Geometry: see drawing. Coordinates: mm, zero at the bounding-box minimum. Coordinates: 2 decimals unless noted, no trailing zeros. Write each loop counter-clockwise with the first axis right and the second up, starting at its lowest first coordinate (ties: lowest second). Pieces come first, ordered by that corner, then holes.
1) Section query A-A (x = 62.5). Output: boundary loops of the cut face in (y, z), then the cut area to 3 significant figures.
2) Section query B-B (y = 1.3). Output: boundary loops of the cut face in (x, z), then the cut area to 3 significant figures.
3) Line query: L1, parallel to Z at x = 89.5, y = 1.2; L2, parallel to X at y = 2.4, z = 71.5; L3, parallel to X at y = 3.95, z = 7.5. Output: solid intervals per line, ascending.
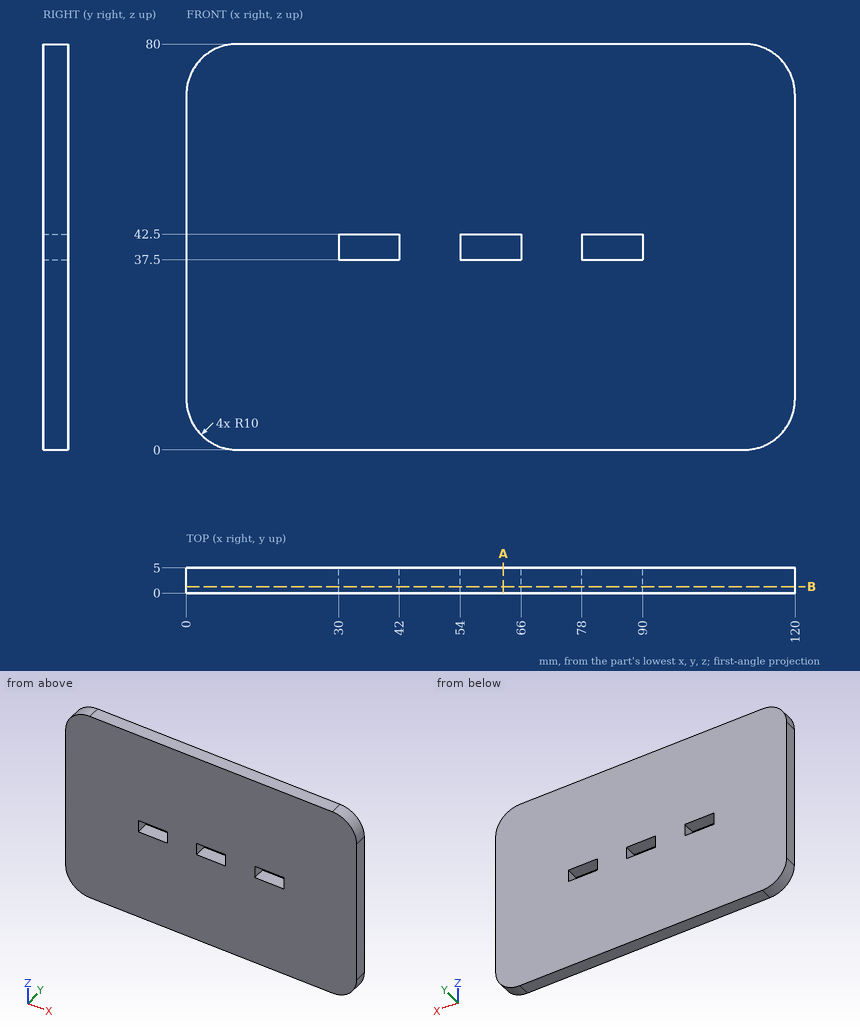
Answer:
1. outline: (0, 0) - (5, 0) - (5, 37.5) - (0, 37.5) - close; (0, 42.5) - (5, 42.5) - (5, 80) - (0, 80) - close
1. area: 375 mm2
2. outline: (0, 10) arc R10 ccw to (10, 0) - (110, 0) arc R10 ccw to (120, 10) - (120, 70) arc R10 ccw to (110, 80) - (10, 80) arc R10 ccw to (0, 70) - close; hole (30, 37.5) - (42, 37.5) - (42, 42.5) - (30, 42.5) - close; hole (54, 37.5) - (66, 37.5) - (66, 42.5) - (54, 42.5) - close; hole (78, 37.5) - (90, 37.5) - (90, 42.5) - (78, 42.5) - close
2. area: 9,330 mm2
3. L1: z = 0 to 37.5, 42.5 to 80
3. L2: x = 0.11 to 119.89
3. L3: x = 0.32 to 119.68
